```python
from build123d import *

# Parameters (mm, degrees)
SKETCH_1_R          = 10
SKETCH_1_R_2        = 4
EXTRUDE_1_DEPTH     = 20
CUT_EXTRUDE_START   = 5
SKETCH_2_R          = 17
CUT_EXTRUDE_1_DEPTH = 10


with BuildPart() as part:
    # 草图1 → 凸台-拉伸1 (new body)
    with BuildSketch(Plane.XY):
        with BuildLine():
            Line((-71.071428571, 14.961685761), (-1.428571429, 19.948914348))
            ThreePointArc((-1.428571429, 19.948914348), (-0.357656609, 19.996801788), (0.714285714, 19.987240828))
            Line((0.714285714, 19.987240828), (140.535714286, 14.990430621))
            ThreePointArc((140.535714286, 14.990430621), (155, 0), (140.535714286, -14.990430621))
            Line((140.535714286, -14.990430621), (0.714285714, -19.987240828))
            ThreePointArc((0.714285714, -19.987240828), (-0.357656609, -19.996801788), (-1.428571429, -19.948914348))
            Line((-1.428571429, -19.948914348), (-71.071428571, -14.961685761))
            ThreePointArc((-71.071428571, -14.961685761), (-85, 0), (-71.071428571, 14.961685761))
        make_face()
        Circle(SKETCH_1_R, mode=Mode.SUBTRACT)
        with Locations((-70, 0)):
            Circle(SKETCH_1_R_2, mode=Mode.SUBTRACT)
        with Locations((140, 0)):
            Circle(SKETCH_1_R_2, mode=Mode.SUBTRACT)
    extrude(amount=EXTRUDE_1_DEPTH)

    # 草图2 → 切除-拉伸1 (cut)
    with BuildSketch(Plane.XY.offset(CUT_EXTRUDE_START)):
        with Locations((140, 0)):
            Circle(SKETCH_2_R)
    extrude(amount=CUT_EXTRUDE_1_DEPTH, mode=Mode.SUBTRACT)


solid = part.part
```
Work out the finished part from the listing and answer in its coordinate system (mm). A direction names the side the tool comes from. Round coordinates to 2 decimals unless told otherwise and drop trailing zeros. Write each loop counter-clockwise with the first axis right and the second up, starting at its lowest first coordinate (ties: lowest second). Pieces come first, ordered by that corner, then holes.
1) Which of the six approach directions +Z, -Z, +X, -X, +Y, -Y give full straight-line access (tool end or side, diameter ignored) to faces 5 (the face through (-66.305, -1.532, 9.86)), 6 (the face through (135, 0, 15))?
2) Consider probe 1 along Y at (x, z) = (140, 3); probe 2 along Y at (x, z) = (0, 5.75); probe 3 along Z at (x, y) = (143, -4). Determine where each line is inside the solid, lowest interval first.
3) A cutting plane is placed at A-A on z = 17.5. Determine the outline of the cut face in (x, y).
4) Flat-ended cylindrical pins translate along their axes: P1, Ø3, axis at x = 91, z = 15, coming from the -Y side; P2, Ø1.5, axis at x = 27, z = 8, coming from the +Y side; P3, Ø5, axis at y = 14, z = 15, coming from the -X side; P4, Ø7, axis at x = -70, y = 0, coming from the +Z side. Find the tip coordinate at first contact, or state that the pin passes through.
5) A cutting plane is placed at C-C on x = -24. Determine the outline of the cut face in (y, z).
6) A cutting plane is placed at D-D on x = 65. Determine the outline of the cut face in (y, z), and give its area (3 significant figures).
7) A cutting plane is placed at B-B on y = 0. Determine the outline of the cut face in (x, z), and give its area (3 significant figures).
8) Determine the mould class of faces 1 (the face through (155, 0, 17)), 2 (the face through (37, 0, 20)), 3 (the face through (-35.76, -17.49, 9.86)), 4 (the face through (143.815, 1.201, 17.465)) for opening direction X: pulls with the +X half, pulls with the -X half, needs draft (parallel to the pull), parting line crosses it, or undercut.
Entries:
1. face 5: +Z, -Z
1. face 6: +X
2. probe 1: y = -15.01 to -4, 4 to 15.01
2. probe 2: y = -20 to -10, 10 to 20
2. probe 3: z = 0 to 5, 15 to 20
3. outline: (-71.07, -14.96) - (-1.43, -19.95) arc R20 ccw to (0.71, -19.99) - (140.54, -14.99) arc R15 ccw to (140.54, 14.99) - (0.71, 19.99) arc R20 ccw to (-1.43, 19.95) - (-71.07, 14.96) arc R15 ccw to start; hole circle Ø8 at (-70, 0); hole circle Ø20 at (0, 0); hole circle Ø8 at (140, 0)
4. P1: stops at y = -16.81
4. P2: stops at y = 19.07
4. P3: stops at x = -79.63
4. P4: passes through
5. outline: (-18.33, 0) - (18.33, 0) - (18.33, 20) - (-18.33, 20) - close
6. outline: (-17.69, 0) - (17.69, 0) - (17.69, 20) - (-17.69, 20) - close
6. area: 708 mm2
7. outline: (-85, 0) - (-74, 0) - (-74, 20) - (-85, 20) - close; (-66, 0) - (-10, 0) - (-10, 20) - (-66, 20) - close; (10, 0) - (136, 0) - (136, 5) - (123, 5) - (123, 15) - (136, 15) - (136, 20) - (10, 20) - close; (144, 0) - (155, 0) - (155, 5) - (144, 5) - close; (144, 15) - (155, 15) - (155, 20) - (144, 20) - close
7. area: 3,840 mm2
8. face 1: pulls with the +X half
8. face 2: needs draft
8. face 3: pulls with the -X half
8. face 4: undercut
